```python
from build123d import *

# Parameters (mm, degrees)
BOSS_EXTRUDE1_DEPTH = 6.35
SKETCH2_R           = 3.3655
CUT_EXTRUDE1_DEPTH  = 7.35
SKETCH3_R           = 2.4638
CUT_EXTRUDE2_DEPTH  = 7.35
SKETCH4_R           = 3.3655
CUT_EXTRUDE3_DEPTH  = 7.35


with BuildPart() as part:
    # Sketch1 → Boss-Extrude1 (new body)
    with BuildSketch(Plane(origin=(0, 0, 0), x_dir=(0, 0, -1), z_dir=(1, 0, 0))):
        Polygon((0, 0), (275.149828585, 365.136155194), (336.005854451, 319.277850429), (296.80346378, 0), align=None)
    extrude(amount=BOSS_EXTRUDE1_DEPTH)

    # Sketch2 → Cut-Extrude1 (cut, through all)
    with BuildSketch(Plane(origin=(6.35, 0, 0), x_dir=(0, 0, -1), z_dir=(1, 0, 0))):
        with Locations((169.042319417, 203.2)):
            Circle(SKETCH2_R)
        with Locations((169.042319417, 184.15)):
            Circle(SKETCH2_R)
        with Locations((169.042319417, 57.15)):
            Circle(SKETCH2_R)
        with Locations((169.042319417, 31.75)):
            Circle(SKETCH2_R)
    extrude(amount=-CUT_EXTRUDE1_DEPTH, mode=Mode.SUBTRACT)

    # Sketch3 → Cut-Extrude2 (cut, through all)
    with BuildSketch(Plane(origin=(6.35, 0, 0), x_dir=(0, 0, -1), z_dir=(1, 0, 0))):
        with Locations((190.5, 30.988)):
            Circle(SKETCH3_R)
        with Locations((190.5, 16.764)):
            Circle(SKETCH3_R)
        with Locations((282.575, 30.988)):
            Circle(SKETCH3_R)
        with Locations((282.575, 16.764)):
            Circle(SKETCH3_R)
        with Locations((285.346343492, 336.461727915)):
            Circle(SKETCH3_R)
        with Locations((276.786126603, 325.10193642)):
            Circle(SKETCH3_R)
    extrude(amount=-CUT_EXTRUDE2_DEPTH, mode=Mode.SUBTRACT)

    # Sketch4 → Cut-Extrude3 (cut, through all)
    with BuildSketch(Plane(origin=(6.35, 0, 0), x_dir=(0, 0, -1), z_dir=(1, 0, 0))):
        with Locations((297.898743163, 316.189372761)):
            Circle(SKETCH4_R)
        with Locations((217.646709826, 209.691327496)):
            Circle(SKETCH4_R)
    extrude(amount=-CUT_EXTRUDE3_DEPTH, mode=Mode.SUBTRACT)


solid = part.part
```
Here's how the part is built. I have some questions about the finished solid (model axes, mm). Coordinates: 2 decimals unless noted, no trailing zeros. Loops run counter-clockwise (first coordinate to the right, second up) from the corner with the lowest first, then second, coordinate; pieces in that order, holes last. Notation, with made-up numbers: (57.25, 57) -> (102.25, 57) arc R23 cw to (102.25, 90) -> close; hole circle Ø5 at (22.5, 2). An arc over 180 degrees is marked (long way). Return JSON: item names as keys, results as strings.
1) Will these pins go through, and if not, where does the flat tip stop? pin 1 (9 mm diameter, centred on y = 209.69, z = -217.65, fed in from +X); pin 2 (3 mm diameter, centred on y = 16.764, z = -282.575, fed in from +X); pin 3 (2 mm diameter, centred on x = 2, z = -66.5, fed in from +Y).
Results below:
{"pin 1": "x = 6.35", "pin 2": "through", "pin 3": "y = 89.58"}
2) If we section it at B-B, the plane z = -39: Write out the boundary of the cut face in (x, y).
Results below:
{"outline": "(0, 0) -> (6.35, 0) -> (6.35, 51.75) -> (0, 51.75) -> close"}
3) I need wall thicknesses on line 1 (Y direction, x = 4, z = -190.5); line 2 (Z direction, x = 2, y = 31); line 3 (Z direction, x = 5.25, y = 56.5). Which ranges of each line are inside material? Lowest first, please. Write a range as from..to.
Results below:
{"line 1": "0..14.3, 19.23..28.52, 33.45..252.8", "line 2": "-300.61..-285.04, -280.11..-192.96, -188.04..-172.32, -165.76..-23.36", "line 3": "-303.74..-172.34, -165.74..-42.58"}
4) If we section it at A-A, the plane x = 1.5: Count the separate pieces of the cut face and the enclosed holes in it, then the cut area to 3 significant figures.
Results below:
{"separate pieces": "1", "enclosed holes": "12", "area": "64,500 mm²"}
5) If we section it at C-C, the plane y = 79: Write out the boundary of the cut face in (x, z), then the cut area to 3 significant figures.
Results below:
{"outline": "(0, -306.5) -> (6.35, -306.5) -> (6.35, -59.53) -> (0, -59.53) -> close", "area": "1,570 mm²"}
